Work out the finished part from the listing and answer in its coordinate system (mm). A direction names the side the tool comes from. Coordinates: 2 decimals unless noted, no trailing zeros. One line per item, written item: value.
```python
from build123d import *

# Parameters (mm, degrees)
F0_R     = 20
F0_R_2   = 18.5078276758
F1_DEPTH = 63.5
F3_R     = 18.6165604835
F3_R_2   = 17.2832490894
F4_DEPTH = 1.27
F6_R     = 20.25
F7_DEPTH = 2


# Not quite as in the source:
# - a fillet or chamfer that OpenCascade refuses, or shapes differently, is made with other operations: its cross-section is extruded or revolved along the edge and cut away or added


with BuildPart() as f1:
    # F0 (on Top) → F1 (new body)
    with BuildSketch(Plane.XY):
        Circle(F0_R)
        Circle(F0_R_2, mode=Mode.SUBTRACT)
    extrude(amount=F1_DEPTH)

    # F2: chamfer of 5.08 x 1.8489687901 on 1 edges, made by hand

    # F2_s1 → F2_t2 (revolve, cut)
    with BuildSketch(Plane.XZ):
        Polygon((20, 5.08), (18.1510312099, 0), (20, 0), align=None)
    revolve(axis=Axis((0, 0, 0), (0, 0, 1)), mode=Mode.SUBTRACT)

    # F3 (on Top) → F4 (join, symmetric)
    with BuildSketch(Plane.XY):
        Circle(F3_R)
        Circle(F3_R_2, mode=Mode.SUBTRACT)
    extrude(amount=F4_DEPTH, both=True)

    # F6 (on offset) → F7 (join)
    with BuildSketch(Plane.XY.offset(-1.2446)):
        Circle(F6_R)
    extrude(amount=-F7_DEPTH)


solid = f1.part
```
Item 1: Given pin 1 (5 mm diameter, centred on x = 3, z = 38, fed in from -Y); pin 2 (5 mm diameter, centred on x = -13.5, z = 25.5, fed in from +Y); pin 3 (8 mm diameter, centred on y = 15.5, z = 25.5, fed in from +X), each flat-ended and moving along its own axis, determine where each tip first touches the part or whether it passes through.
Evaluation:
pin 1: stops at y = -19.99
pin 2: stops at y = 16.7
pin 3: stops at x = 16.36
Item 2: Determine the mould class of faces 4 (the face through (6, -18, 63.5)), 5 (the face through (11, 17, -2)), 6 (the face through (5, 17, 1.27)) for opening direction X: +X half, -X half, draft (parallel to the pull), parting line (faces both ways), or undercut.
Evaluation:
face 4: draft
face 5: parting line
face 6: undercut
Item 3: Consider probe 1 along Y at (x, z) = (0, 0); probe 2 along Z at (x, y) = (17, 0.5); probe 3 along X at (y, z) = (-11, 1.5). Determine where each line is inside the solid, lowest interval first.
Evaluation:
probe 1: y = -18.62 to -17.28, 17.28 to 18.62
probe 2: z = -3.24 to -1.24
probe 3: x = -15.12 to -14.88, 14.88 to 15.12
Item 4: Which of the six approach directions +Z, -Z, +X, -X, +Y, -Y give full straight-line access (tool end or side, diameter ignored) to faces 1 (the face through (16.485, 5.191, -0.005)), 2 (the face through (0, 0, -3.245)), 3 (the face through (18, -6, -1.245))?
Evaluation:
face 1: +Z
face 2: -Z, +X, -X, +Y, -Y
face 3: none
